```python
from build123d import *

# Parameters (mm, degrees)
F1_DEPTH = 63.5
F2_W     = 63.5
F2_H     = 50.8
F3_DEPTH = 25.4
F4_W     = 29.5556526983
F4_H     = 38.1
F5_DEPTH = 50.8


with BuildPart() as f1:
    # F0 (on Front) → F1 (new body)
    with BuildSketch(Plane.XZ):
        Polygon((-59.3443473017, 44.5968605516), (-59.3443473017, 19.1968605516), (-21.2443494164, 19.1968605516), (-21.2443494164, -31.6031394484), (54.9556526983, -31.6031394484), (54.9556526983, -6.2031394484), (4.1556526983, -6.2031394484), (4.1556526983, 44.5968605516), align=None)
    extrude(amount=-F1_DEPTH)

    # F2 (on face) → F3 (join)
    with BuildSketch(Plane.YZ.offset(4.1556526983)):
        with Locations((31.75, 19.1968605516)):
            Rectangle(F2_W, F2_H)
    extrude(amount=F3_DEPTH)

    # F4 (on face) → F5 (cut)
    with BuildSketch(Plane.XY.offset(44.5968605516)):
        with Locations((14.7778263491, 19.05)):
            Rectangle(F4_W, F4_H)
    extrude(amount=-F5_DEPTH, mode=Mode.SUBTRACT)


solid = f1.part
```
CAD build for the part. Positions are in the model's coordinates, mm. A direction names the side the tool comes from. Round coordinates to 2 decimals unless told otherwise and drop trailing zeros. Order: outer loops, then holes, each group sorted by start corner. A loop starts at its lowest first (then second) coordinate and runs counter-clockwise, first axis right, second up.
Q1. Slice it at C-C (x = 9). Write the cut outline in (y, z).
Q2. Slice it at A-A (y = 52.5). Write the cut outline in (x, z).
Q3. Which spindle directions (+Z, -Z, +X, -X, +Y, -Y) get a long thin tool onto all of the face, cutting with end or side? Do faces 4 (the flat face through (0, 19, 20)), 5 (the flat face through (-3, 0, 6)), 6 (the flat face through (-21.244, 31, -6)). Say none if no direction does.
Q4. Two-plate mould, pull along Z, no slides. Class faces 1 (the flat face through (16, 31, -31.603)), 2 (the flat face through (-25, 31, 44.597)), 3 (the flat face through (29.556, 51, 20)): pulls with the +Z half, pulls with the -Z half, needs draft (parallel to the pull), parting line crosses it, or undercut.
Q5. Wall check: L1, parallel to X at y = 51, z = 41; L2, parallel to X at y = 26, z = -6.5; L3, parallel to Z at x = -38, y = 46. Give the ranges that are in metal, low to high.
Q6. Drop flat-ended pins along their axis: pin 1 (15 mm diameter, centred on x = 9.5, z = 28.5, fed in from -Y); pin 2 (20.5 mm diameter, centred on y = 50.5, z = 21, fed in from +X); pin 3 (12 mm diameter, centred on y = 34, z = 0, fed in from -X). Give the stop position or say it passes through.
Q7. Slice it at D-D (y = 9). Write the cut outline in (x, z).
Q8. Slice it at B-B (z = 10.5). Write the cut outline in (x, y).
Results below:
1. outline: (0, -31.6) - (63.5, -31.6) - (63.5, 44.6) - (38.1, 44.6) - (38.1, -6.2) - (0, -6.2) - close
2. outline: (-59.34, 19.2) - (-21.24, 19.2) - (-21.24, -31.6) - (54.96, -31.6) - (54.96, -6.2) - (29.56, -6.2) - (29.56, 44.6) - (-59.34, 44.6) - close
3. face 4: +Z, +X, -Y
3. face 5: +Z, -Z, +X, -X, -Y
3. face 6: -Z, -X, +Y, -Y
4. face 1: pulls with the -Z half
4. face 2: pulls with the +Z half
4. face 3: needs draft
5. L1: x = -59.34 to 29.56
5. L2: x = -21.24 to 54.96
5. L3: z = 19.2 to 44.6
6. pin 1: stops at y = 38.1
6. pin 2: stops at x = 29.56
6. pin 3: stops at x = -21.24
7. outline: (-59.34, 19.2) - (-21.24, 19.2) - (-21.24, -31.6) - (54.96, -31.6) - (54.96, -6.2) - (0, -6.2) - (0, 44.6) - (-59.34, 44.6) - close
8. outline: (-21.24, 0) - (0, 0) - (0, 38.1) - (29.56, 38.1) - (29.56, 63.5) - (-21.24, 63.5) - close
